```python
from build123d import *

# Parameters (mm, degrees)
BOSS_EXTRUDE1_START     = -15.24
BOSS_EXTRUDE1_DEPTH     = 12.192
CUT_EXTRUDE4_DEPTH      = 6.35
CUT_EXTRUDE4_DEPTH_BACK = 8.89
SKETCH4_R               = 2.0955


with BuildPart() as part:
    # Sketch1 → Revolve1 (revolve)
    with BuildSketch(Plane(origin=(0, 0, 0), x_dir=(1, 0, 0), z_dir=(0, 1, 0))):
        Polygon((2.54, 6.35), (2.54, -6.35), (2.54, -8.89), (5.08, -8.89), (5.08, -31.75), (7.62, -31.75), (7.62, -6.35), (5.08, -6.35), (5.08, 6.35), align=None)
    revolve(axis=Axis((0, 0, 6.35), (0, 0, -1)))

    # Sketch2 → Boss-Extrude1 (add)
    with BuildSketch(Plane(origin=(0, 0, -6.35), x_dir=(-1, 0, 0), z_dir=(0, 0, -1)).offset(BOSS_EXTRUDE1_START)):
        with BuildLine():
            Line((1.651, -1.930232888), (1.651, 1.930232888))
            ThreePointArc((1.651, 1.930232888), (2.54, 0), (1.651, -1.930232888))
        make_face()
        with BuildLine():
            Line((-1.651, -1.930232888), (-1.651, 1.930232888))
            ThreePointArc((-1.651, 1.930232888), (-2.54, 0), (-1.651, -1.930232888))
        make_face()
    extrude(amount=BOSS_EXTRUDE1_DEPTH)

    # Sketch4 → Cut-Extrude4 (cut, two sides: drawn at the far end of the back side and taken through both)
    with BuildSketch(Plane(origin=(0, 0, 0), x_dir=(0, 0, -1), z_dir=(1, 0, 0)).offset(-CUT_EXTRUDE4_DEPTH_BACK)):
        with Locations(Location((-25.4, 0, 0), (0, 0, 180))):
            Circle(SKETCH4_R)
    extrude(amount=CUT_EXTRUDE4_DEPTH + CUT_EXTRUDE4_DEPTH_BACK, mode=Mode.SUBTRACT)


solid = part.part
```
For this review, take the finished solid that the model builds, in its own axes (mm). A direction names the side the tool comes from. Round coordinates to 2 decimals unless told otherwise and drop trailing zeros. Order: outer loops, then holes, each group sorted by start corner. A loop starts at its lowest first (then second) coordinate and runs counter-clockwise, first axis right, second up.
Q1. Wall thickness on line 1 (X direction, y = 0, z = 14.25); line 2 (Y direction, x = 0, z = -2.25); line 3 (X direction, y = 0, z = 1): over which ranges is each line inside the solid? List them lowest first.
Findings below:
line 1: x = -7.62 to -5.08, 5.08 to 7.62
line 2: y = -5.08 to -2.54, 2.54 to 5.08
line 3: x = -5.08 to -1.65, 1.65 to 5.08
Q2. Insertion check: P1, Ø5, axis at x = -6, z = 15.5, coming from the +Y side; P2, Ø3, axis at x = 2, y = 2.5, coming from the +Z side; P3, Ø4.5, axis at x = 0, y = 0, coming from the -Z side. Each pin has a flat end and moves straight along its axis. Give the tip position at first contact, or say it passes through.
Findings below:
P1: stops at y = 6.77
P2: stops at z = 8.89
P3: stops at z = -3.3
Q3. We need section A-A, the plane x = 0. Give the boundary of the cut face in (y, z).
Findings below:
outline: (-7.62, 6.35) - (-5.08, 6.35) - (-5.08, -6.35) - (-2.54, -6.35) - (-2.54, 8.89) - (-5.08, 8.89) - (-5.08, 31.75) - (-7.62, 31.75) - close; (2.54, -6.35) - (5.08, -6.35) - (5.08, 6.35) - (7.62, 6.35) - (7.62, 31.75) - (5.08, 31.75) - (5.08, 8.89) - (2.54, 8.89) - close
Q4. We need section C-C, the plane z = 20. Give the boundary of the cut face in (x, y).
Findings below:
outline: circle Ø15.24 at (0, 0); hole circle Ø10.16 at (0, 0)
Q5. Machinability: for faces 5 (the cylindrical face through (5.67, -1.42, 23.86)), 6 (the flat face through (-2, 5, 31.75)), 7 (the cylindrical face through (-5.075, -0.223, 20.48)), 8 (the flat face through (-1.651, 0, 3)), 9 (the cylindrical face through (1.172, 2.253, -0.317)), which of the approach directions +Z, -Z, +X, -X, +Y, -Y give a long, thin tool a straight path to every point of the face, cutting with its end or side? Answer none if there is none.
Findings below:
face 5: -X
face 6: +Z, +X, -X, +Y, -Y
face 7: +Z
face 8: +Z, -Z
face 9: -Z
Q6. We need section D-D, the plane y = 3. Give the boundary of the cut face in (x, z), plus the area to 3 significant figures.
Findings below:
outline: (-7, 6.35) - (-4.1, 6.35) - (-4.1, -6.35) - (4.1, -6.35) - (4.1, 6.35) - (7, 6.35) - (7, 31.75) - (4.1, 31.75) - (4.1, 8.89) - (-4.1, 8.89) - (-4.1, 31.75) - (-7, 31.75) - close
area: 273 mm2
Q7. We need section B-B, the plane y = 0. Give the boundary of the cut face in (x, z).
Findings below:
outline: (-7.62, 6.35) - (-5.08, 6.35) - (-5.08, -6.35) - (-2.54, -6.35) - (-2.54, -3.3) - (-1.65, -3.3) - (-1.65, 8.89) - (-5.08, 8.89) - (-5.08, 23.3) - (-7.62, 23.3) - close; (-7.62, 27.5) - (-5.08, 27.5) - (-5.08, 31.75) - (-7.62, 31.75) - close; (1.65, -3.3) - (2.54, -3.3) - (2.54, -6.35) - (5.08, -6.35) - (5.08, 6.35) - (7.62, 6.35) - (7.62, 31.75) - (5.08, 31.75) - (5.08, 27.5) - (6.35, 27.5) - (6.35, 23.3) - (5.08, 23.3) - (5.08, 8.89) - (1.65, 8.89) - close
Q8. Mouldability with a two-part tool opening along X and no side actions: class faces 1 (the flat face through (2, 5, 6.35)), 2 (the flat face through (-2, 0, 8.89)), 3 (the flat face through (2, 0, -3.302)), 4 (the cylindrical face through (-0.661, -5.037, -0.089)) as pulls with the +X half, pulls with the -X half, needs draft (parallel to the pull), parting line crosses it, or undercut.
Findings below:
face 1: needs draft
face 2: undercut
face 3: undercut
face 4: parting line crosses it
